Verification items for the finished model (mm, model axes). A direction names the side the tool comes from. Give positions to 0.01 mm unless a question says otherwise; leave off trailing zeros. Write each loop counter-clockwise with the first axis right and the second up, starting at its lowest first coordinate (ties: lowest second). Pieces come first, ordered by that corner, then holes.
from build123d import *

# Parameters (mm, degrees)
SKETCH_1_R               = 12
EXTRUDE_1_DEPTH          = 4
SKETCH_2_R               = 5
EXTRUDE_2_DEPTH          = 20
CHAMFER_1_SIZE           = 0.4
CUT_EXTRUDE_1_DEPTH      = 30.393876913
CUT_EXTRUDE_1_DEPTH_BACK = 30.393876913
SKETCH_4_R               = 1.45
CHAMFER_2_SIZE           = 1.5


with BuildPart() as part:
    # 草图1 → 凸台-拉伸1 (new body)
    with BuildSketch(Plane(origin=(0, 0, 0), x_dir=(1, 0, 0), z_dir=(0, 1, 0))):
        with Locations(Location((0, 0, 0), (0, 0, 270))):
            Circle(SKETCH_1_R)
    extrude(amount=EXTRUDE_1_DEPTH)

    # 草图2 → 凸台-拉伸2 (add)
    with BuildSketch(Plane(origin=(0, 4, 0), x_dir=(1, 0, 0), z_dir=(0, 1, 0))):
        with Locations(Location((0, 0, 0), (0, 0, 270))):
            Circle(SKETCH_2_R)
    extrude(amount=EXTRUDE_2_DEPTH)

    # 倒角1
    chamfer_1_edges = [part.edges().sort_by_distance(p)[0] for p in [
        (0, 4, -12),
        (0, 24, -5),
    ]]
    chamfer(chamfer_1_edges, length=CHAMFER_1_SIZE)

    # 草图4 → 切除-拉伸1 (cut, two sides: drawn at the far end of the back side and taken through both)
    with BuildSketch(Plane(origin=(0, 0, 0), x_dir=(0, 0, -1), z_dir=(1, 0, 0)).offset(-CUT_EXTRUDE_1_DEPTH_BACK)):
        with Locations(Location((0, 20, 0), (0, 0, 180))):
            Circle(SKETCH_4_R)
    extrude(amount=CUT_EXTRUDE_1_DEPTH + CUT_EXTRUDE_1_DEPTH_BACK, mode=Mode.SUBTRACT)

    # 倒角2
    chamfer_2_edges = [part.edges().sort_by_distance(p)[0] for p in [
        (0, 4, -5),
    ]]
    chamfer(chamfer_2_edges, length=CHAMFER_2_SIZE)


solid = part.part
Item 1: Depth check by flat-ended pin: pin 1 (3 mm diameter, centred on x = -4, y = 7, fed in from +Z); pin 2 (4 mm diameter, centred on x = 4.5, y = 3.5, fed in from -Z); pin 3 (12 mm diameter, centred on x = -0.5, y = 12, fed in from -Z); pin 4 (6 mm diameter, centred on y = 20, z = 8.5, fed in from +X). Enter the tip coordinate at first touch or a pass-through.
Answer key:
pin 1: stops at z = 4.33
pin 2: stops at z = -11.74
pin 3: stops at z = -5
pin 4: passes through
Item 2: Sectioned sample at A-A on x = 0. Record the cut outline in (y, z), then the cut area to 3 significant figures.
Answer key:
outline: (0, -12) - (3.6, -12) - (4, -11.6) - (4, -6.5) - (5.5, -5) - (23.6, -5) - (24, -4.6) - (24, 4.6) - (23.6, 5) - (5.5, 5) - (4, 6.5) - (4, 11.6) - (3.6, 12) - (0, 12) - close; hole circle Ø2.9 at (20, 0)
area: 291 mm2
Item 3: Sectioned sample at D-D on y = 20. Record the cut outline in (x, z).
Answer key:
outline: (-4.79, -1.45) arc R5 ccw to (4.79, -1.45) - close; (-4.79, 1.45) - (4.79, 1.45) arc R5 ccw to start
Item 4: Sectioned sample at B-B on z = 0. Record the cut outline in (x, y).
Answer key:
outline: (-12, 0) - (12, 0) - (12, 3.6) - (11.6, 4) - (6.5, 4) - (5, 5.5) - (5, 18.55) - (-5, 18.55) - (-5, 5.5) - (-6.5, 4) - (-11.6, 4) - (-12, 3.6) - close; (-5, 21.45) - (5, 21.45) - (5, 23.6) - (4.6, 24) - (-4.6, 24) - (-5, 23.6) - close
Item 5: Scan lines: line 1 along Y through (x, z) = (-1.75, 0); line 2 along Y through (x, z) = (8.75, 3.5); line 3 along Z through (x, y) = (-2.5, 21). Record each from-to range of solid material in increasing order.
Answer key:
line 1: y = 0 to 18.55, 21.45 to 24
line 2: y = 0 to 4
line 3: z = -4.33 to -1.05, 1.05 to 4.33
Item 6: Set-up check for faces 1 (the face through (-5, 4, 5)), 2 (the face through (-0.07, 21.416, -0.314)): record each of +Z, -Z, +X, -X, +Y, -Y from which the full face is reachable in a straight line by a thin tool's end or side.
Answer key:
face 1: +Y
face 2: +X, -X
Item 7: Sectioned sample at C-C on y = 6.5. Record the cut outline in (x, z), then the cut area to 3 significant figures.
Answer key:
outline: circle Ø10 at (0, 0)
area: 78.5 mm2
